Here's the drawing with two shaded views (mm, measured from the low corner). I have some questions. A direction names the side the tool comes from. Coordinates: 2 decimals unless noted, no trailing zeros. Write each loop counter-clockwise with the first axis right and the second up, starting at its lowest first coordinate (ties: lowest second). Pieces come first, ordered by that corner, then holes.
Item 1: I want a section at C-C on x = 5.5. Please give me the cut outline in (y, z).
Item 2: I want a section at D-D on z = 8. Please give me the cut outline in (x, y).
Item 3: Thinking about a two-plate mould opening in X: for the marked faces 4, 5 and 6, which applies, +X half, -X half, draft (parallel to the pull), parting line (faces both ways), or undercut?
Item 4: Which directions (+Z, -Z, +X, -X, +Y, -Y) give clear straight access to the entire face, cutting with the end or side of a thin tool? Please do the marked faces 1, 2 and 3.
Item 5: If I drill on probe 1 along X at (y, z) = (14, 16); probe 2 along Z at (x, y) = (16.5, 8); probe 3 along Y at (x, z) = (22, 5), over which ranges is the centre line in solid material (lowest first)?
Item 6: I want a section at A-A on x = 16. Please give me the cut outline in (y, z), then the cut area to 3 significant figures.
Item 7: I want a section at B-B on y = 37.5. Please give me the cut outline in (x, z).
Item 8: For P1, Ø2, axis at y = 12.5, z = 12.5, coming from the -X side; P2, Ø2, axis at x = 23.5, y = 50, coming from the -Z side; P3, Ø3, axis at x = 14.5, y = 9, coming from the +Z side; P4, Ø16, axis at y = 60, z = 21, coming from the -X side, each with a flat end and sliding along its axis, tell me the tip position at first contact or that it passes through.
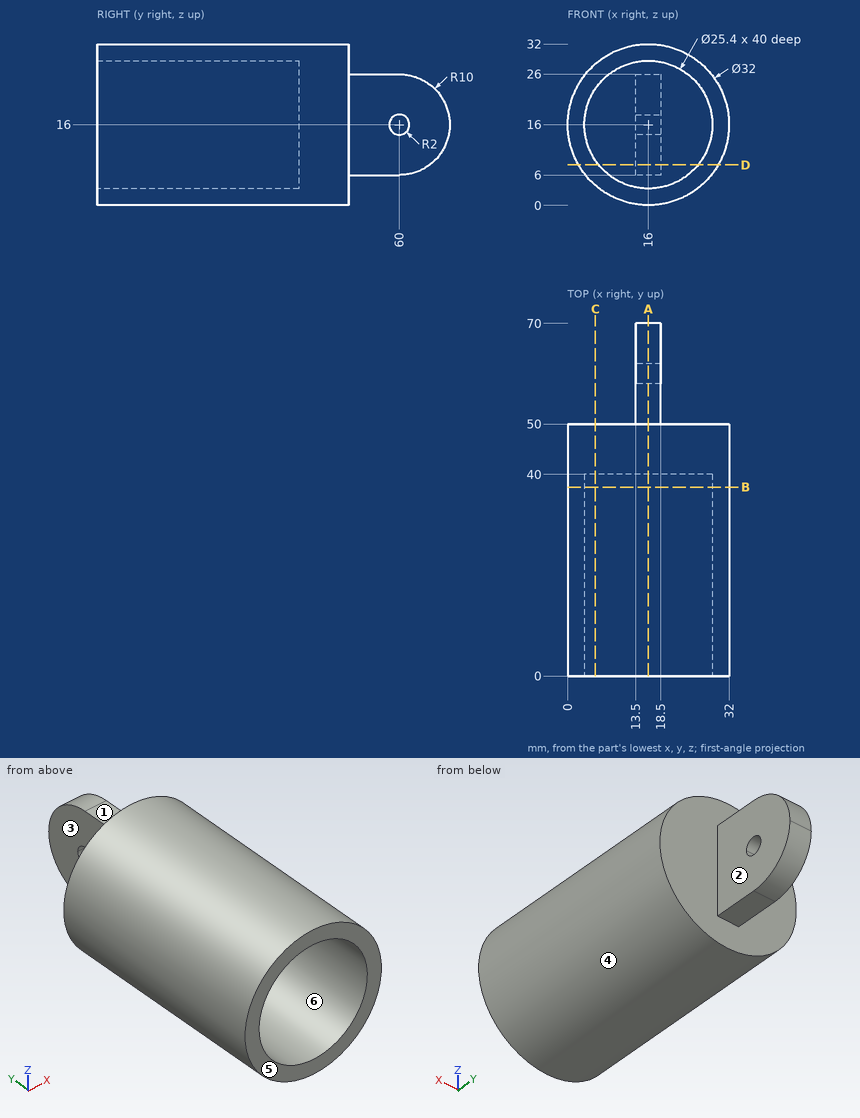
Response values:
1. outline: (0, 3.93) - (50, 3.93) - (50, 28.07) - (0, 28.07) - (0, 23.14) - (40, 23.14) - (40, 8.86) - (0, 8.86) - close
2. outline: (2.14, 0) - (6.14, 0) - (6.14, 40) - (25.86, 40) - (25.86, 0) - (29.86, 0) - (29.86, 50) - (18.5, 50) - (18.5, 66) - (13.5, 66) - (13.5, 50) - (2.14, 50) - close
3. face 4: parting line
3. face 5: draft
3. face 6: undercut
4. face 1: +Z, +X, -X, +Y
4. face 2: +Z, -Z, +X, +Y
4. face 3: +Z, -Z, -X, +Y
5. probe 1: x = 0 to 3.3, 28.7 to 32
5. probe 2: z = 0.01 to 3.31, 28.69 to 31.99
5. probe 3: y = 40 to 50
6. outline: (0, 0) - (50, 0) - (50, 6) - (60, 6) arc R10 ccw to (60, 26) - (50, 26) - (50, 32) - (0, 32) - (0, 28.7) - (40, 28.7) - (40, 3.3) - (0, 3.3) - close; hole circle Ø4 at (60, 16)
6. area: 929 mm2
7. outline: circle Ø32 at (16, 16); hole circle Ø25.4 at (16, 16)
8. P1: stops at x = 0.2
8. P2: stops at z = 1.38
8. P3: stops at z = 32
8. P4: stops at x = 13.5
